Can you work these out from the model? Positions are in its coordinate system, mm. A direction names the side the tool comes from. Give positions to 0.01 mm unless a question says otherwise; leave off trailing zeros. Write each loop counter-clockwise with the first axis right and the second up, starting at its lowest first coordinate (ties: lowest second). Pieces come first, ordered by that corner, then holes.
```python
from build123d import *

# Parameters (mm, degrees)
F0_W     = 49
F0_H     = 28
F0_R     = 2.5
F1_DEPTH = 3
F0_W_2   = 3
F0_H_2   = 2
F2_DEPTH = 60
F4_DEPTH = 55
F5_W     = 13
F5_H     = 19
F5_R     = 2
F6_DEPTH = 25


# Not quite as in the source:
# - a feature names something its author has since deleted; it is built from what else it names


with BuildPart() as f1:
    # F0 (on Top) → F1 (new body)
    with BuildSketch(Plane.XY):
        with Locations((0, 1)):
            Rectangle(F0_W, F0_H)
        with Locations((-17.5, 0)):
            Circle(F0_R, mode=Mode.SUBTRACT)
        with Locations((17.5, 0)):
            Circle(F0_R, mode=Mode.SUBTRACT)
    extrude(amount=F1_DEPTH)

    # F0 (on Top) → F2 (join)
    with BuildSketch(Plane.XY):
        with Locations((-26, 1)):
            Rectangle(F0_W_2, F0_H)
        with Locations((-26, -14)):
            Rectangle(F0_W_2, F0_H_2)
        with Locations((0, -14)):
            Rectangle(F0_W, F0_H_2)
        with Locations((26, -14)):
            Rectangle(F0_W_2, F0_H_2)
        with Locations((26, 1)):
            Rectangle(F0_W_2, F0_H)
    extrude(amount=F2_DEPTH)

    # F3 (on face) → F4 (cut)
    with BuildSketch(Plane(origin=(-27.5, 0, 0), x_dir=(0, -1, 0), z_dir=(-1, 0, 0))):
        Polygon((13, 60), (-15, 60), (-15, 3), align=None)
    extrude(amount=-F4_DEPTH, mode=Mode.SUBTRACT)

    # F5 (on face) → F6 (cut)
    with BuildSketch(Plane.XZ.offset(15)):
        Polygon((-22.5, 53), (-22.5, 36), (-9.5, 36), (-9.5, 55), (-22.5, 55), align=None)
        with Locations((-16, 19.5)):
            Rectangle(F5_W, F5_H)
        with Locations((0.5, 19.5)):
            Circle(F5_R)
        with Locations((17.5, 19.5)):
            Circle(F5_R)
    extrude(amount=-F6_DEPTH, mode=Mode.SUBTRACT)


solid = f1.part
```
1) If we mould it in two halves opening along Z, with no side actions, what happens to faces 1 (the face through (-22.5, -14, 46)), 2 (the face through (-24.5, -2, 25)), 3 (the face through (0, 0, 0)), 4 (the face through (-16, -14, 10))? For each: +Z half, -Z half, draft (parallel to the pull), parting line (faces both ways), or undercut.
Values follow:
face 1: undercut
face 2: draft
face 3: -Z half
face 4: undercut
2) Suppose I cut it at C-C on x = 17.5. Write out the boundary of the cut face in (y, z), plus the area to 3 significant figures.
Values follow:
outline: (-15, 0) - (-2.5, 0) - (-2.5, 3) - (-13, 3) - (-13, 17.5) - (-15, 17.5) - close; (-15, 21.5) - (-13, 21.5) - (-13, 60) - (-15, 60) - close; (2.5, 0) - (15, 0) - (15, 3) - (2.5, 3) - close
area: 181 mm2
3) Suppose I cut it at D-D on z = 42.5. Write out the boundary of the cut face in (x, y), plus the area to 3 significant figures.
Values follow:
outline: (-27.5, -15) - (-22.5, -15) - (-22.5, -13) - (-24.5, -13) - (-24.5, -4.4) - (-27.5, -4.4) - close; (-9.5, -15) - (27.5, -15) - (27.5, -4.4) - (24.5, -4.4) - (24.5, -13) - (-9.5, -13) - close
area: 136 mm2
4) For faces 5 (the face through (24.5, -2, 25)), 6 (the face through (-16, -14, 55)), 7 (the face through (0, -14, 60)), which set-ups out of +Z, -Z, +X, -X, +Y, -Y let a thin tool reach every point of the face, with its end or its side?
Values follow:
face 5: +Z, +Y
face 6: +Y, -Y
face 7: +Z, +X, -X, +Y, -Y
5) Suppose I cut it at A-A on x = 0.5. Write out the boundary of the cut face in (y, z), plus the area to 3 significant figures.
Values follow:
outline: (-15, 0) - (15, 0) - (15, 3) - (-13, 3) - (-13, 17.5) - (-15, 17.5) - close; (-15, 21.5) - (-13, 21.5) - (-13, 60) - (-15, 60) - close
area: 196 mm2
6) Suppose I cut it at B-B on x = -17.5. Write out the boundary of the cut face in (y, z), plus the area to 3 significant figures.
Values follow:
outline: (-15, 0) - (-2.5, 0) - (-2.5, 3) - (-13, 3) - (-13, 10) - (-15, 10) - close; (-15, 29) - (-13, 29) - (-13, 36) - (-15, 36) - close; (-15, 55) - (-13, 55) - (-13, 60) - (-15, 60) - close; (2.5, 0) - (15, 0) - (15, 3) - (2.5, 3) - close
area: 113 mm2
7) For pin 1 Ø1 at (x, z) = (-8.5, 34) entering from +Y; pin 2 Ø10 at (x, y) = (-2.5, -6) entering from +Z, each with a flat end and sliding along its axis, tell me the tip position at first contact or that it passes through.
Values follow:
pin 1: stops at y = -13
pin 2: stops at z = 3
8) Please list where these lines run through material, in increasing order: L1, parallel to Z at x = 17.5, y = -13.5; L2, parallel to Y at x = 17.5, z = 0.7; L3, parallel to X at y = -3.75, z = 24.5.
Values follow:
L1: z = 0 to 17.5, 21.5 to 60
L2: y = -15 to -2.5, 2.5 to 15
L3: x = -27.5 to -24.5, 24.5 to 27.5
